```python
from build123d import *

# Parameters (mm, degrees)
SKETCH1_W           = 55.560809748
SKETCH1_H           = 22
SKETCH1_R           = 1.5
BOSS_EXTRUDE1_DEPTH = 2
SKETCH3_R           = 2.5
CUT_EXTRUDE1_DEPTH  = 2


with BuildPart() as part:
    # Sketch1 → Boss-Extrude1 (new body)
    # profile 1 of 4: a face of its own
    with BuildSketch(Plane.XY):
        Polygon((-62.402927025, 55.272853248), (-46.347522151, 32.642853248), (-22.897522151, 32.642853248), (88.224097345, 32.642853248), (104.279502219, 55.272853248), (48.718692471, 55.272853248), (-6.842117277, 55.272853248), align=None)
    # profile 2 of 4: a face of its own
    with BuildSketch(Plane.XY):
        with Locations((-34.622522151, 66.272853248)):
            Rectangle(SKETCH1_W, SKETCH1_H)
        with Locations((-55.512724588, 67.272853248)):
            Circle(SKETCH1_R, mode=Mode.SUBTRACT)
        with Locations((-13.732319714, 67.272853248)):
            Circle(SKETCH1_R, mode=Mode.SUBTRACT)
    # profile 3 of 4: a face of its own
    with BuildSketch(Plane.XY):
        with Locations((20.938287597, 66.272853248)):
            Rectangle(SKETCH1_W, SKETCH1_H)
        with Locations((0.04808516, 67.272853248)):
            Circle(SKETCH1_R, mode=Mode.SUBTRACT)
        with Locations((41.828490034, 67.272853248)):
            Circle(SKETCH1_R, mode=Mode.SUBTRACT)
    # profile 4 of 4: a face of its own
    with BuildSketch(Plane.XY):
        with Locations((76.499097345, 66.272853248)):
            Rectangle(SKETCH1_W, SKETCH1_H)
        with Locations((55.608894908, 67.272853248)):
            Circle(SKETCH1_R, mode=Mode.SUBTRACT)
        with Locations((97.389299782, 67.272853248)):
            Circle(SKETCH1_R, mode=Mode.SUBTRACT)
    extrude(amount=BOSS_EXTRUDE1_DEPTH)

    # Sketch3 → Cut-Extrude1 (cut)
    with BuildSketch(Plane(origin=(0, 0, 0), x_dir=(-1, 0, 0), z_dir=(0, 0, -1))):
        with Locations((-48.718692471, 42.642853248)):
            Circle(SKETCH3_R)
        with Locations(Location((6.842117277, 42.642853248, 0), (0, 0, 180))):
            Circle(SKETCH3_R)
    extrude(amount=-CUT_EXTRUDE1_DEPTH, mode=Mode.SUBTRACT)


solid = part.part
```
CAD build for the part. Positions are in the model's coordinates, mm. Coordinates: 2 decimals unless noted, no trailing zeros. Write each loop counter-clockwise with the first axis right and the second up, starting at its lowest first coordinate (ties: lowest second). Pieces come first, ordered by that corner, then holes. Notation, with made-up numbers: (25, -33) -> (52, -33) arc R7 ccw to (52, -27) -> close; hole circle Ø5 at (-32, 8). An arc over 180 degrees is marked (long way). Return JSON: item names as keys, results as strings. Group by question number.
Q1. Flat gauge pin, fed straight in: pin 1 (4 mm diameter, centred on x = -6.84, y = 42.64, fed in from -Z). Where does the tip first touch, or does it go through?
Q2. Cut at B-B, the plane y = 52. Give the cut face in (x, z), then the cut area to 3 significant figures.
Q3. Drill centre lines: line 1 (X direction, y = 43, z = 0.35); line 2 (Y direction, x = 47, z = 1.4); line 3 (Y direction, x = -15, z = 0.45). Where is each one in solid material? Low to high.
Q4. Cut at A-A, the plane z = 0.9. State how many separate pieces and enclosed holes the cut face has, then the cut area to 3 significant figures.
Q5. Pull direction X, two halves, no side cores. Call faces 1 (the face through (-4.46, 41.89, 0.99)), 2 (the face through (-54.49, 44.12, 0.99)), 3 (the face through (20, 55, 0)): released by +X, released by -X, zero draft, split by the parting line, or undercut.
Returned:
{
 "1": {"pin 1": "passes through"},
 "2": {"outline": "(-60.08, 0) -> (101.96, 0) -> (101.96, 2) -> (-60.08, 2) -> close", "area": "324 mm2"},
 "3": {"line 1": "x = -53.7 to -9.32, -4.37 to 46.24, 51.19 to 95.57", "line 2": "y = 32.64 to 40.83, 44.46 to 77.27", "line 3": "y = 32.64 to 66.47, 68.07 to 77.27"},
 "4": {"separate pieces": "1", "enclosed holes": "8", "area": "6,990 mm2"},
 "5": {"face 1": "undercut", "face 2": "released by -X", "face 3": "zero draft"}
}
